CAD build for the part. Positions are in the model's coordinates, mm. Round coordinates to 2 decimals unless told otherwise and drop trailing zeros. Order: outer loops, then holes, each group sorted by start corner. A loop starts at its lowest first (then second) coordinate and runs counter-clockwise, first axis right, second up. Notation, with made-up numbers: (32, -24.5) - (81, -24.5) arc R18 ccw to (81, 3.5) - close; hole circle Ø4 at (69.25, 19.25). An arc over 180 degrees is marked (long way). Use one line per item in the form item = value. Start each with the question number.
from build123d import *

# Parameters (mm, degrees)
SKETCH_1_W          = 100
SKETCH_1_H          = 100
EXTRUDE_1_DEPTH     = 2
SKETCH_2_R          = 1.6
CUT_EXTRUDE_1_DEPTH = 2
SKETCH_3_R          = 1.6
CUT_EXTRUDE_2_DEPTH = 10
SKETCH_4_R          = 6
CUT_EXTRUDE_3_DEPTH = 38.65
SKETCH_5_R          = 1.6
CUT_EXTRUDE_4_DEPTH = 38.6
SKETCH_6_R          = 1.6
CUT_EXTRUDE_5_DEPTH = 10


with BuildPart() as part:
    # ｽｹｯﾁ1 → ﾎﾞｽ - 押し出し1 (new body)
    with BuildSketch(Plane.XY):
        Rectangle(SKETCH_1_W, SKETCH_1_H)
    extrude(amount=EXTRUDE_1_DEPTH)

    # ｽｹｯﾁ2 → ｶｯﾄ - 押し出し1 (cut)
    with BuildSketch(Plane.XY.offset(2)):
        with Locations((-45, 42.5)):
            Circle(SKETCH_2_R)
        with Locations((-25, 42.5)):
            Circle(SKETCH_2_R)
        with Locations((25, 42.5)):
            Circle(SKETCH_2_R)
        with Locations((45, 42.5)):
            Circle(SKETCH_2_R)
    extrude(amount=-CUT_EXTRUDE_1_DEPTH, mode=Mode.SUBTRACT)

    # ｽｹｯﾁ3 → ｶｯﾄ - 押し出し2 (cut)
    with BuildSketch(Plane.XY.offset(2)):
        with Locations((0, -41)):
            Circle(SKETCH_3_R)
    extrude(amount=-CUT_EXTRUDE_2_DEPTH, mode=Mode.SUBTRACT)

    # ｽｹｯﾁ4 → ｶｯﾄ - 押し出し3 (cut)
    with BuildSketch(Plane.XY.offset(2)):
        with Locations((-18.25, 19)):
            Circle(SKETCH_4_R)
        with Locations((18.25, 19)):
            Circle(SKETCH_4_R)
    extrude(amount=-CUT_EXTRUDE_3_DEPTH, mode=Mode.SUBTRACT)

    # ｽｹｯﾁ5 → ｶｯﾄ - 押し出し4 (cut)
    with BuildSketch(Plane.XY.offset(2)):
        with Locations((-18.25, -11)):
            Circle(SKETCH_5_R)
        with Locations((18.25, -11)):
            Circle(SKETCH_5_R)
    extrude(amount=-CUT_EXTRUDE_4_DEPTH, mode=Mode.SUBTRACT)

    # ｽｹｯﾁ6 → ｶｯﾄ - 押し出し5 (cut)
    with BuildSketch(Plane.XY.offset(2)):
        with Locations((-39.3, -41)):
            Circle(SKETCH_6_R)
        with Locations((39.3, -41)):
            Circle(SKETCH_6_R)
    extrude(amount=-CUT_EXTRUDE_5_DEPTH, mode=Mode.SUBTRACT)


solid = part.part
(1) Slice it at A-A (x = 0). Give the cut face in (y, z).
(2) Wall check: line 1 (Y direction, x = -18.25, z = 1.15); line 2 (Y direction, x = 45, z = 1.5); line 3 (X direction, y = 15, z = 0.2). Give the ranges that are in metal, low to high. Write a range as [from, to].
(3) Slice it at C-C (z = 1.2). Give the number of separate pieces and of enclosed holes in the cut face, and give its area (3 significant figures).
(4) Flat gauge pins, fed straight in: P1, Ø5, axis at x = -39.3, y = -41, coming from the -Z side; P2, Ø3, axis at x = 18.25, y = -11, coming from the -Z side. Where does each tip first touch, or does it go through?
(5) Mould opens along X. For faces 1 (the cylindrical face through (-23.01, 15.35, 1.01)), 2 (the flat face through (-1, 1, 0)) say: pulls with the +X half, pulls with the -X half, needs draft (parallel to the pull), parting line crosses it, or undercut.
(6) Slice it at B-B (y = -41). Give the cut face in (x, z), and give its area (3 significant figures).
(7) Slice it at D-D (y = 19). Give the cut face in (x, z).
Results list:
q1.outline = (-50, 0) - (-42.6, 0) - (-42.6, 2) - (-50, 2) - close; (-39.4, 0) - (50, 0) - (50, 2) - (-39.4, 2) - close
q2.line_1 = [-50, -12.6], [-9.4, 13], [25, 50]
q2.line_2 = [-50, 40.9], [44.1, 50]
q2.line_3 = [-50, -22.72], [-13.78, 13.78], [22.72, 50]
q3.separate_pieces = 1
q3.enclosed_holes = 11
q3.area = 9,700 mm²
q4.P1 = 0
q4.P2 = through
q5.face_1 = undercut
q5.face_2 = needs draft
q6.outline = (-50, 0) - (-40.9, 0) - (-40.9, 2) - (-50, 2) - close; (-37.7, 0) - (-1.6, 0) - (-1.6, 2) - (-37.7, 2) - close; (1.6, 0) - (37.7, 0) - (37.7, 2) - (1.6, 2) - close; (40.9, 0) - (50, 0) - (50, 2) - (40.9, 2) - close
q6.area = 181 mm²
q7.outline = (-50, 0) - (-24.25, 0) - (-24.25, 2) - (-50, 2) - close; (-12.25, 0) - (12.25, 0) - (12.25, 2) - (-12.25, 2) - close; (24.25, 0) - (50, 0) - (50, 2) - (24.25, 2) - close
